from build123d import *

# Parameters (mm, degrees)
SKETCH1_W       = 8.73125
SKETCH1_H       = 8.73125
EXTRUDE1_DEPTH  = 3.175
LPATTERN2_COUNT = 5
LPATTERN2_PITCH = 0.79375
CHAMFER1_SIZE   = 0.396875
CHAMFER1_SIZE_2 = 0.290532664


with BuildPart() as part:
    # Sketch1 → Extrude1 (new body)
    with BuildSketch(Plane(origin=(0, 0, 0), x_dir=(1, 0, 0), z_dir=(0, 1, 0))):
        Rectangle(SKETCH1_W, SKETCH1_H)
    extrude(amount=EXTRUDE1_DEPTH)

    # Sketch2 → Cut-Revolve1 (revolve, cut)
    with BuildSketch(Plane.XY, mode=Mode.PRIVATE) as cut_revolve1_sk:
        Polygon((0, 3.175), (1.65317021, 3.175), (2.0828, 2.926953125), (2.0828, 2.827734375), (1.65317021, 2.5796875), (1.65317021, 2.38125), (0, 2.38125), align=None)
    cut_revolve1 = revolve(cut_revolve1_sk.sketch.rotate(Axis((0, 1.663578541, 0), (0, -1, 0)), 90), axis=Axis((0, 1.663578541, 0), (0, -1, 0)), mode=Mode.SUBTRACT)

    # LPattern2: Cut-Revolve1 ×5
    with Locations(*[(0, -i * LPATTERN2_PITCH, 0) for i in range(1, LPATTERN2_COUNT)]):
        add(cut_revolve1, mode=Mode.SUBTRACT)

    # Chamfer1
    # the kernel refuses this chamfer: 0.396875, 0.290532664 mm, written as the material it takes off along each edge
    with BuildSketch(Plane(origin=(0, 3.175, 0), x_dir=(0, 0, 1), z_dir=(1, 0, 0))) as chamfer1_piece_1:
        Polygon((1.65317021 + CHAMFER1_SIZE, 0), (1.65317021 + CHAMFER1_SIZE_2 * 0.866025404541, CHAMFER1_SIZE_2 * 0.500000000437), (1.65317021, 0), align=None)
    revolve(axis=Axis((0, 3.175, 0), (0, -1, 0)), mode=Mode.SUBTRACT)


solid = part.part
The listing builds one solid part. Answer for the finished solid, in the listing's coordinates (mm). Coordinates: 2 decimals unless noted, no trailing zeros. Write each loop counter-clockwise with the first axis right and the second up, starting at its lowest first coordinate (ties: lowest second). Pieces come first, ordered by that corner, then holes. Notation, with made-up numbers: (38, 52) -> (92, 52) arc R13 cw to (92, 65) -> close; hole circle Ø10 at (14.5, 68.25). An arc over 180 degrees is marked (long way). One line per question, with ' | ' between items.
1. Section A-A (y = 2.7) is taken. Determine the outline of the cut face in (x, z).
Verdict:
outline: (-4.37, -4.37) -> (4.37, -4.37) -> (4.37, 4.37) -> (-4.37, 4.37) -> close; hole circle Ø3.72 at (0, 0)
2. Given pin 1 Ø3 at (x, z) = (0, 0) entering from -Y, flat-ended and moving along its own axis, determine where the tip first touches the part or whether it passes through.
Verdict:
pin 1: passes through
3. Straight lines are drawn through the part: line 1 (X direction, y = 1.7, z = 0); line 2 (X direction, y = 0.5, z = 0); line 3 (Z direction, x = 1.25, y = 1.85). For each, find the intervals that lie inside material, in ascending order.
Verdict:
line 1: x = -4.37 to -1.65, 1.65 to 4.37 | line 2: x = -4.37 to -2.08, 2.08 to 4.37 | line 3: z = -4.37 to -1.24, 1.24 to 4.37
